from build123d import *

# Parameters (mm, degrees)
SKETCH_1_R               = 2.5
EXTRUDE_1_DEPTH          = 46.35
M3X0_5_1_D               = 2.5
M3X0_5_1_DEPTH           = 8.5
M3X0_5_1_TIP             = 0.751075774
M3X0_5_1_ON_FACE_2_D     = 2.5
M3X0_5_1_ON_FACE_2_DEPTH = 8.5
M3X0_5_1_ON_FACE_2_TIP   = 0.751075774


with BuildPart() as part:
    # ｽｹｯﾁ1 → ﾎﾞｽ - 押し出し1 (new body, symmetric)
    with BuildSketch(Plane.XY):
        Circle(SKETCH_1_R)
    extrude(amount=EXTRUDE_1_DEPTH, both=True)

    # M3x0.5 ねじ穴1
    with Locations(Plane.XY.offset(46.35)):
        with Locations((0, 0)):
            Hole(M3X0_5_1_D / 2, depth=M3X0_5_1_DEPTH)
            with Locations((0, 0, -(M3X0_5_1_DEPTH + M3X0_5_1_TIP / 2))):  # 118° drill point
                Cone(0, M3X0_5_1_D / 2, M3X0_5_1_TIP, mode=Mode.SUBTRACT)

    # M3x0.5 ねじ穴1 on face 2
    with Locations(Plane(origin=(0, 0, -46.35), x_dir=(-1, 0, 0), z_dir=(0, 0, -1))):
        with Locations((0, 0)):
            Hole(M3X0_5_1_ON_FACE_2_D / 2, depth=M3X0_5_1_ON_FACE_2_DEPTH)
            with Locations((0, 0, -(M3X0_5_1_ON_FACE_2_DEPTH + M3X0_5_1_ON_FACE_2_TIP / 2))):  # 118° drill point
                Cone(0, M3X0_5_1_ON_FACE_2_D / 2, M3X0_5_1_ON_FACE_2_TIP, mode=Mode.SUBTRACT)


solid = part.part
Check sheet for the modelled part. Datum: model origin and axes. Units: mm. A direction names the side the tool comes from. Round coordinates to 2 decimals unless told otherwise and drop trailing zeros. Order: outer loops, then holes, each group sorted by start corner. A loop starts at its lowest first (then second) coordinate and runs counter-clockwise, first axis right, second up. Notation, with made-up numbers: M 48,55 L 90,55 A13 cw 90,59 Z; hole C 75,85.25 d3. An arc over 180 degrees is marked long. One line per item, written item: value. Start each with the question number.
1. Access from +Z, -Z, +X, -X, +Y, -Y to the whole of each face (thin tool, end or side, straight path). Record for faces 1 (the cylindrical face through (-0.27, -1.22, -42.04)), 2 (the cylindrical face through (0.27, -1.22, 42.04)), 3 (the flat face through (-1, -1, -46.35)).
2. Section check A-A on z = -30. Enter the section's corners in (x, y).
3. Scan lines: line 1 along Y through (x, z) = (0, 44.5); line 2 along X through (y, z) = (0.1, 19.5). Record each from-to range of solid material in increasing order.
4. Release check for a two-part mould opening along Y. For faces 4 (the cylindrical face through (-0.54, -2.44, 0.65)), 5 (the conical face through (0.05, -0.21, -37.23)), 6 (the conical face through (-0.05, -0.21, 37.23)), 7 (the flat face through (-1, -1, 46.35)) record: released by +Y, released by -Y, zero draft, split by the parting line, or undercut.
5. Gauge pin test, flat ends, axial feed: P1, Ø2, axis at x = 0, y = 0, coming from the +Z side; P2, Ø2, axis at y = 1.5, z = -13.5, coming from the -X side. Record the tip position at first contact, or that the pin passes through.
Results found:
1. face 1: -Z
1. face 2: +Z
1. face 3: -Z, +X, -X, +Y, -Y
2. outline: C 0,0 d5
3. line 1: -2.5 to -1.25, 1.25 to 2.5
3. line 2: -2.5 to 2.5
4. face 4: split by the parting line
4. face 5: undercut
4. face 6: undercut
4. face 7: zero draft
5. P1: z = 37.7
5. P2: x = -2.45
